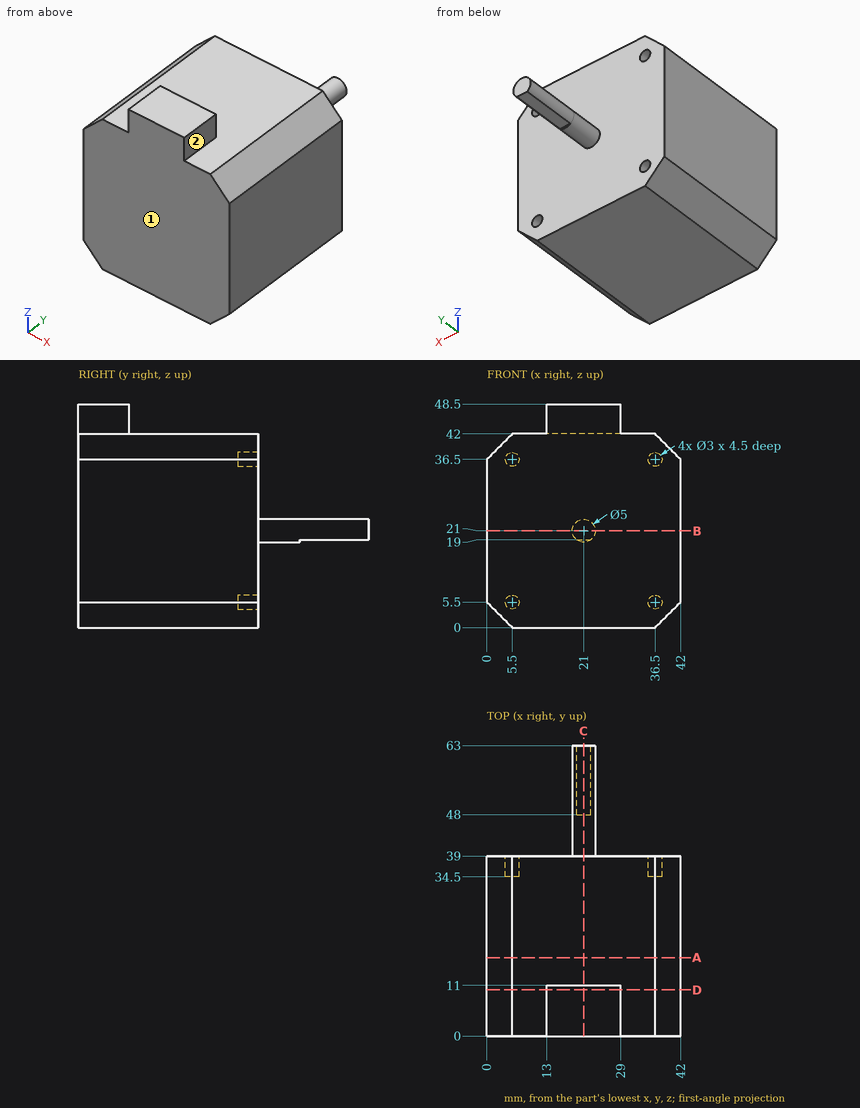
Input: dimensioned drawing with shaded views. Units: mm. Origin: part minimum x, y, z. A direction names the side the tool comes from. Coordinates: 2 decimals unless noted, no trailing zeros. Order: outer loops, then holes, each group sorted by start corner. A loop starts at its lowest first (then second) coordinate and runs counter-clockwise, first axis right, second up. Notation, with made-up numbers: (33, -13.5) -> (55, -13.5) arc R12 ccw to (55, 1.5) -> close; hole circle Ø2 at (21, 39). An arc over 180 degrees is marked (long way). Answer in a Markdown table with one row per item.
Item 1: Section B-B on z = 21. Output: boundary loops of the cut face in (x, y), plus the area to 3 significant figures.
Return value:
| item | result |
|---|---|
| outline | (0, 0) -> (42, 0) -> (42, 39) -> (23.5, 39) -> (23.5, 63) -> (18.5, 63) -> (18.5, 39) -> (0, 39) -> close |
| area | 1,760 mm² |
Item 2: Ray query, L1, parallel to X at y = 36.2, z = 36.5; L2, parallel to Z at x = 36, y = 36; L3, parallel to Y at x = 39.5, z = 30.5. Return the intervals inside material, ascending.
Return value:
| item | result |
|---|---|
| L1 | x = 0 to 4, 7 to 35, 38 to 42 |
| L2 | z = 0 to 4.09, 6.91 to 35.09, 37.91 to 42 |
| L3 | y = 0 to 39 |
Item 3: Access query for the marked faces 1 and 2. Directions: +Z, -Z, +X, -X, +Y, -Y. A direction counts if a zero-diameter tool reaches every point of the face in a straight line with its end or side. Return the directions, or none.
Return value:
| item | result |
|---|---|
| face 1 | +Z, -Z, +X, -X, -Y |
| face 2 | +Z, +X, +Y, -Y |
Item 4: Contact query for flat-ended pins moving along their axis: P1, Ø7, axis at x = 22.5, z = 44.5, coming from the +Y side; P2, Ø0.9, axis at x = 5, z = 37, coming from the +Y side; P3, Ø2, axis at y = 4, z = 44.5, coming from the -X side. Output: stop coordinate, or through.
Return value:
| item | result |
|---|---|
| P1 | stops at y = 39 |
| P2 | stops at y = 34.5 |
| P3 | stops at x = 13 |
Item 5: Section C-C on x = 21. Output: boundary loops of the cut face in (y, z).
Return value:
| item | result |
|---|---|
| outline | (0, 0) -> (39, 0) -> (39, 18.5) -> (48, 18.5) -> (48, 19) -> (63, 19) -> (63, 23.5) -> (39, 23.5) -> (39, 42) -> (11, 42) -> (11, 48.5) -> (0, 48.5) -> close |
Item 6: Section A-A on y = 17. Output: boundary loops of the cut face in (x, z), plus the area to 3 significant figures.
Return value:
| item | result |
|---|---|
| outline | (0, 5.5) -> (5.5, 0) -> (36.5, 0) -> (42, 5.5) -> (42, 36.5) -> (36.5, 42) -> (5.5, 42) -> (0, 36.5) -> close |
| area | 1,700 mm² |
Item 7: Section D-D on y = 10. Output: boundary loops of the cut face in (x, z).
Return value:
| item | result |
|---|---|
| outline | (0, 5.5) -> (5.5, 0) -> (36.5, 0) -> (42, 5.5) -> (42, 36.5) -> (36.5, 42) -> (29, 42) -> (29, 48.5) -> (13, 48.5) -> (13, 42) -> (5.5, 42) -> (0, 36.5) -> close |
